Build history of the part. All positions in model axes, mm. Face numbers are marked on the shaded views. Round coordinates to 2 decimals unless told otherwise and drop trailing zeros. Write each loop counter-clockwise with the first axis right and the second up, starting at its lowest first coordinate (ties: lowest second). Pieces come first, ordered by that corner, then holes. Notation, with made-up numbers: (18, 1.25) - (38, 1.25) arc R14 ccw to (38, 14.25) - close; hole circle Ø1 at (0.25, -15). An arc over 180 degrees is marked (long way). Answer as a JSON object with one key per item and string values. Group by question number.
Item 1: Probe line 1 (Y direction, x = 39.6, z = 0.75); line 2 (Y direction, x = -32.4, z = 1); line 3 (Y direction, x = -40, z = 2.75). List the from-to ranges inside material, lowest first. Write a range as from..to.
Item 2: Slice it at C-C, the plane y = -2.75. List the corners of the cut face in (x, z), then the cut area to 3 significant figures.
Item 3: Flat gauge pins, fed straight in: pin 1 (1 mm diameter, centred on x = -8.5, y = 5.5, fed in from -Z); pin 2 (1 mm diameter, centred on y = 3.5, z = 3, fed in from -X); pin 3 (2.5 mm diameter, centred on x = 17, y = 3, fed in from +Z); pin 4 (1.8 mm diameter, centred on x = -9.5, z = 3.5, fed in from -Y). Where does each tip first touch, or does it go through?
Item 4: Two-plate mould, pull along X, no slides. Class the marked faces 1 and 2: +X half, -X half, draft (parallel to the pull), parting line (faces both ways), or undercut.
Item 5: Slice it at B-B, the plane z = 3.75. List the corners of the cut face in (x, y), then the cut area to 3 significant figures.
Item 6: Slice it at A-A, the plane x = -32.4. List the corners of the cut face in (y, z).
Item 7: Slice it at D-D, the plane x = 26.2. List the corners of the cut face in (y, z), then the cut area to 3 significant figures.
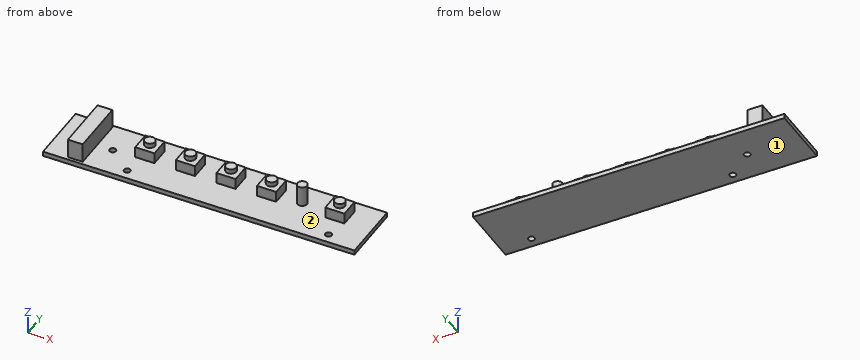
from build123d import *

# Parameters (mm, degrees)
F0_W      = 99
F0_H      = 19.8
F1_DEPTH  = 1.5
F2_W      = 6.1
F2_H      = 6.1
F3_DEPTH  = 3.5
F4_R      = 1.65
F5_DEPTH  = 1.5
F6_R      = 1.5
F7_DEPTH  = 6.5
F8_W      = 4.7
F8_H      = 18
F9_DEPTH  = 6.2
F10_R     = 1
F11_DEPTH = 1.501


with BuildPart() as f1:
    # F0 (on Top) → F1 (new body)
    with BuildSketch(Plane.XY):
        Rectangle(F0_W, F0_H)
    extrude(amount=F1_DEPTH)

    # F2 (on face) → F3 (join)
    with BuildSketch(Plane.XY.offset(1.5)):
        with Locations((38.15, 2.95)):
            Rectangle(F2_W, F2_H)
        with Locations((16.45, 2.95)):
            Rectangle(F2_W, F2_H)
        with Locations((3.55, 2.95)):
            Rectangle(F2_W, F2_H)
        with Locations((-9.35, 2.95)):
            Rectangle(F2_W, F2_H)
        with Locations((-22.25, 2.95)):
            Rectangle(F2_W, F2_H)
    extrude(amount=F3_DEPTH)

    # F4 (on face) → F5 (join)
    with BuildSketch(Plane.XY.offset(5)):
        with Locations((-22.25, 2.95)):
            Circle(F4_R)
        with Locations((-9.35, 2.95)):
            Circle(F4_R)
        with Locations((3.55, 2.95)):
            Circle(F4_R)
        with Locations((16.45, 2.95)):
            Circle(F4_R)
        with Locations((38.15, 2.95)):
            Circle(F4_R)
    extrude(amount=F5_DEPTH)

    # F6 (on face) → F7 (join)
    with BuildSketch(Plane.XY.offset(1.5)):
        with Locations((26.2, 2.95)):
            Circle(F6_R)
    extrude(amount=F7_DEPTH)

    # F8 (on face) → F9 (join)
    with BuildSketch(Plane.XY.offset(1.5)):
        with Locations((-39.75, 0.1)):
            Rectangle(F8_W, F8_H)
    extrude(amount=F9_DEPTH)

    # F10 (on face) → F11 (cut, through all)
    with BuildSketch(Plane.XY.offset(1.5)):
        with Locations((-24.4, -6.7)):
            Circle(F10_R)
        with Locations((-32.4, -0.2)):
            Circle(F10_R)
        with Locations((39.6, -6.7)):
            Circle(F10_R)
    extrude(amount=-F11_DEPTH, mode=Mode.SUBTRACT)


solid = f1.part
Geometry says:
{
 "1": {"line 1": "y = -9.9..-7.7, -5.7..9.9", "line 2": "y = -9.9..-1.2, 0.8..9.9", "line 3": "y = -8.9..9.1"},
 "2": {"outline": "(-49.5, 0) - (49.5, 0) - (49.5, 1.5) - (-37.4, 1.5) - (-37.4, 7.7) - (-42.1, 7.7) - (-42.1, 1.5) - (-49.5, 1.5) - close", "area": "178 mm^2"},
 "3": {"pin 1": "stops at z = 0", "pin 2": "stops at x = -42.1", "pin 3": "stops at z = 6.5", "pin 4": "stops at y = -0.1"},
 "4": {"face 1": "draft", "face 2": "undercut"},
 "5": {"outline": "(-42.1, -8.9) - (-37.4, -8.9) - (-37.4, 9.1) - (-42.1, 9.1) - close; (-25.3, -0.1) - (-19.2, -0.1) - (-19.2, 6) - (-25.3, 6) - close; (-12.4, -0.1) - (-6.3, -0.1) - (-6.3, 6) - (-12.4, 6) - close; (0.5, -0.1) - (6.6, -0.1) - (6.6, 6) - (0.5, 6) - close; (13.4, -0.1) - (19.5, -0.1) - (19.5, 6) - (13.4, 6) - close; circle Ø3 at (26.2, 2.95); (35.1, -0.1) - (41.2, -0.1) - (41.2, 6) - (35.1, 6) - close", "area": "278 mm^2"},
 "6": {"outline": "(-9.9, 0) - (-1.2, 0) - (-1.2, 1.5) - (-9.9, 1.5) - close; (0.8, 0) - (9.9, 0) - (9.9, 1.5) - (0.8, 1.5) - close"},
 "7": {"outline": "(-9.9, 0) - (9.9, 0) - (9.9, 1.5) - (4.45, 1.5) - (4.45, 8) - (1.45, 8) - (1.45, 1.5) - (-9.9, 1.5) - close", "area": "49.2 mm^2"}
}
